Job drawing, mm, ordinate dimensions from the low corner. One solid piece. Give positions to 0.01 mm unless a question says otherwise; leave off trailing zeros. Write each loop counter-clockwise with the first axis right and the second up, starting at its lowest first coordinate (ties: lowest second). Pieces come first, ordered by that corner, then holes. Notation, with made-up numbers: M 0,22 L 49,22 A15 cw 49,39 Z; hole C 20.25,47 d11. An arc over 180 degrees is marked long. Use a Markdown table: item, result.
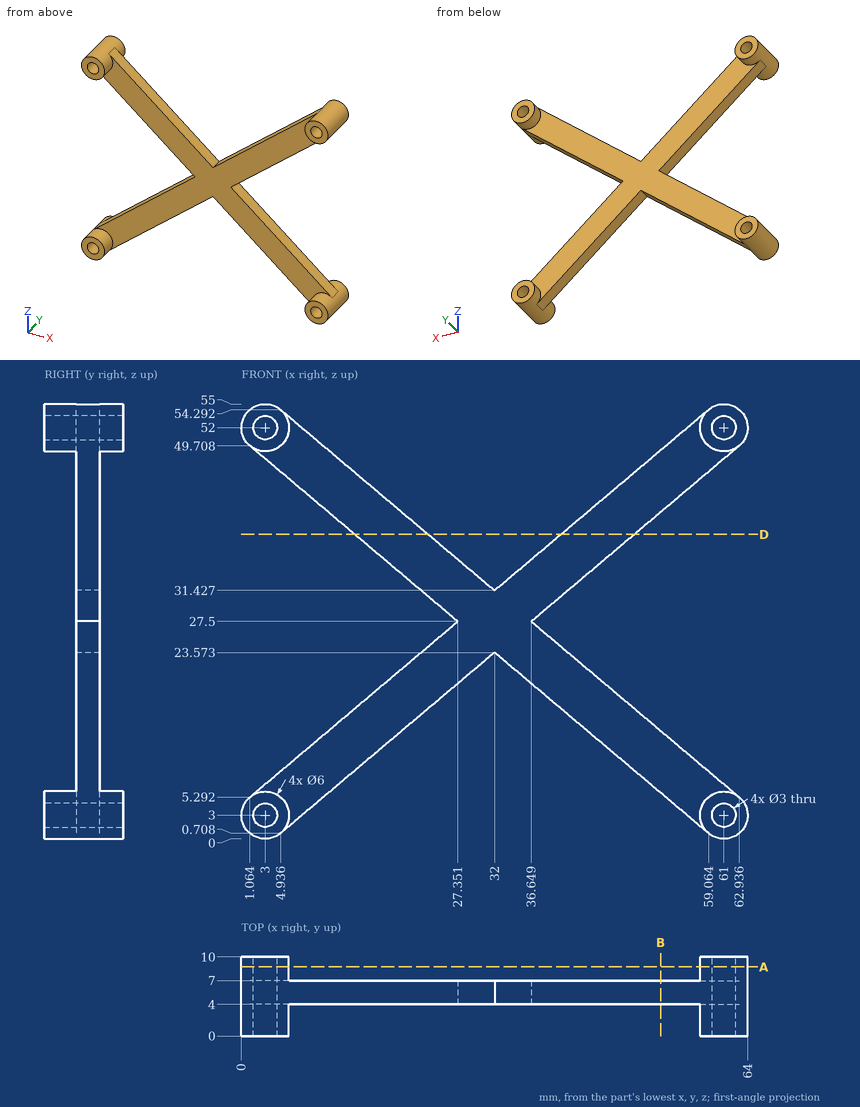
1. Drill centre lines: L1, parallel to X at y = 2, z = 3; L2, parallel to X at y = 4.5, z = 3; L3, parallel to Z at x = 26, y = 6.25 (1 decimal). Where is each one in solid material? Low to high.
Findings below:
| item | result |
|---|---|
| L1 | 0 to 1.5, 4.5 to 6, 58 to 59.5, 62.5 to 64 |
| L2 | 0 to 1.5, 4.5 to 7.65, 56.35 to 59.5, 62.5 to 64 |
| L3 | 18.5 to 26.4, 28.6 to 36.5 |
2. Cut at D-D, the plane z = 38.5. Give the cut face in (x, y).
Findings below:
| item | result |
|---|---|
| outline | M 14.33,4 L 23.63,4 L 23.63,7 L 14.33,7 Z; M 40.37,4 L 49.67,4 L 49.67,7 L 40.37,7 Z |
3. Drop flat-ended pins along their axis: P1, Ø2, axis at y = 6, z = 46, coming from the +X side; P2, Ø2, axis at y = 2.5, z = 48.5, coming from the +X side; P3, Ø1, axis at x = 49.5, y = 7, coming from the +Z side (1 decimal). Give the stop position or say it passes through.
Findings below:
| item | result |
|---|---|
| P1 | x = 59.73 |
| P2 | x = 62.66 |
| P3 | z = 46.6 |
4. Cut at B-B, the plane x = 53. Give the cut face in (y, z).
Findings below:
| item | result |
|---|---|
| outline | M 4,5.83 L 7,5.83 L 7,13.69 L 4,13.69 Z; M 4,41.31 L 7,41.31 L 7,49.17 L 4,49.17 Z |
5. Cut at A-A, the plane y = 8.75. Give the cut face in (x, z).
Findings below:
| item | result |
|---|---|
| outline | C 3,3 d6; C 3,52 d6; C 61,3 d6; C 61,52 d6; hole C 3,3 d3; hole C 3,52 d3; hole C 61,3 d3; hole C 61,52 d3 |
